```python
from build123d import *

# Parameters (mm, degrees)
SKETCH1_R           = 15
BOSS_EXTRUDE1_DEPTH = 130
CHAMFER1_SIZE       = 2
SKETCH2_W           = 1.6
SKETCH2_H           = 0.7


with BuildPart() as part:
    # Sketch1 → Boss-Extrude1 (new body)
    with BuildSketch(Plane.XY):
        Circle(SKETCH1_R)
    extrude(amount=BOSS_EXTRUDE1_DEPTH)

    # Chamfer1
    chamfer1_edges = [part.edges().sort_by_distance(p)[0] for p in [
        (-15, 0, 0),
        (-15, 0, 130),
    ]]
    chamfer(chamfer1_edges, length=CHAMFER1_SIZE)

    # Sketch2 → Cut-Revolve1 (revolve, cut)
    with BuildSketch(Plane(origin=(0, 0, 0), x_dir=(0, 0, -1), z_dir=(1, 0, 0)), mode=Mode.PRIVATE) as cut_revolve1_sk:
        with Locations((-125.2, 14.65)):
            Rectangle(SKETCH2_W, SKETCH2_H)
        with Locations((-4.8, 14.65)):
            Rectangle(SKETCH2_W, SKETCH2_H)
    revolve(cut_revolve1_sk.sketch.rotate(Axis((0, 0, 130), (0, 0, -1)), 90), axis=Axis((0, 0, 130), (0, 0, -1)), mode=Mode.SUBTRACT)


solid = part.part
```
Input: part model. Units: mm. Frame: model coordinates. A direction names the side the tool comes from. Coordinates: 2 decimals unless noted, no trailing zeros. Loops run counter-clockwise (first coordinate to the right, second up) from the corner with the lowest first, then second, coordinate; pieces in that order, holes last. Notation, with made-up numbers: (56.25, -24) - (85.25, -24) arc R26 ccw to (85.25, 15) - close; hole circle Ø8 at (-10, 21). An arc over 180 degrees is marked (long way). Answer in a Markdown table with one row per item.
(1) Material intervals for L1, parallel to X at y = -0.75, z = 100; L2, parallel to Y at x = -7.5, z = 95.5; L3, parallel to X at y = 6, z = 62, sorted ascending. Write a range as from..to.
Model answer:
| item | result |
|---|---|
| L1 | x = -14.98..14.98 |
| L2 | y = -12.99..12.99 |
| L3 | x = -13.75..13.75 |
(2) Pin query (flat end, axial travel): P1, Ø2, axis at y = -3.5, z = 28, coming from the -X side; P2, Ø1.5, axis at y = -8, z = 78, coming from the +X side; P3, Ø3, axis at x = 2.5, z = 30, coming from the -Y side. Return the tip coordinate at first contact, or that it passes through.
Model answer:
| item | result |
|---|---|
| P1 | stops at x = -14.79 |
| P2 | stops at x = 13.13 |
| P3 | stops at y = -14.97 |
(3) Cut plane A-A on z = 81. Output: boundary loops of the cut face in (x, y), plus the area to 3 significant figures.
Model answer:
| item | result |
|---|---|
| outline | circle Ø30 at (0, 0) |
| area | 707 mm² |
(4) Mould query, pull axis Z, two halves, no side actions, for faces 1 (the face through (0, 0, 0)), 2 (the face through (-1.86, -14.18, 125.19)), 3 (the face through (0, 0, 130)), 4 (the face through (-14.985, 0.66, 126.986)). Classes: pulls with the +Z half, pulls with the -Z half, needs draft (parallel to the pull), parting line crosses it, or undercut.
Model answer:
| item | result |
|---|---|
| face 1 | pulls with the -Z half |
| face 2 | undercut |
| face 3 | pulls with the +Z half |
| face 4 | needs draft |
(5) Set-up query: faces 5 (the face through (-1.86, -14.18, 4.79)), 6 (the face through (-14.985, 0.66, 64.168)). Return all of +Z, -Z, +X, -X, +Y, -Y with unobstructed straight access to the full face (end or side cutting, diameter ignored); none if empty.
Model answer:
| item | result |
|---|---|
| face 5 | none |
| face 6 | +Z, -Z |
